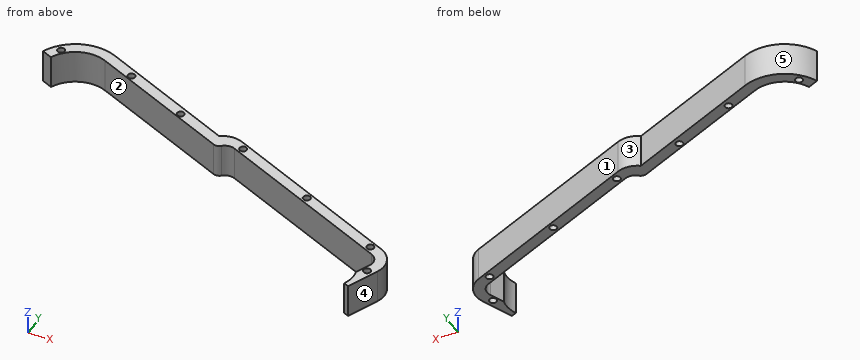
```python
from build123d import *

# Parameters (mm, degrees)
SKETCH1_R           = 14.25
SKETCH1_R_2         = 1.7
SKETCH1_R_3         = 1.6
BOSS_EXTRUDE1_DEPTH = 15
SKETCH5_R           = 1.25
SKETCH5_R_2         = 1.6
CUT_EXTRUDE4_DEPTH  = 16
CUT_EXTRUDE5_DEPTH  = 16
FILLET1_R           = 5
FILLET2_R           = 5
CUT_EXTRUDE6_DEPTH  = 16
CUT_EXTRUDE7_DEPTH  = 16
FILLET5_R           = 3
SKETCH9_R           = 14
CUT_EXTRUDE8_DEPTH  = 16


with BuildPart() as part:
    # Sketch1 → Boss-Extrude1 (new body)
    with BuildSketch(Plane.XY):
        with BuildLine():
            Line((-72.715301765, 90.837326721), (-152.817002247, 126.544575004))
            ThreePointArc((-152.817002247, 126.544575004), (-157.784388135, 127.370762315), (-162.524605276, 125.671394934))
            Line((-162.524605276, 125.671394934), (-222.299360222, 152.317421212))
            ThreePointArc((-222.299360222, 152.317421212), (-249.039738928, 142.066706765), (-238.78902448, 115.326328059))
            Line((-238.78902448, 115.326328059), (-179.014269534, 88.680301782))
            ThreePointArc((-179.014269534, 88.680301782), (-177.109561802, 84.018800254), (-173.174612442, 80.876558766))
            Line((-173.174612442, 80.876558766), (-93.072911961, 45.169310483))
            ThreePointArc((-93.072911961, 45.169310483), (-85.421957972, 44.965480094), (-79.867786674, 50.231391692))
            Line((-79.867786674, 50.231391692), (-67.653220557, 77.632201435))
            ThreePointArc((-67.653220557, 77.632201435), (-67.449390168, 85.283155423), (-72.715301765, 90.837326721))
        make_face()
        with Locations((-230.544192351, 133.821874636)):
            Circle(SKETCH1_R, mode=Mode.SUBTRACT)
        with Locations((-95.571468701, 49.02024728)):
            Circle(SKETCH1_R_2, mode=Mode.SUBTRACT)
        with Locations((-132.105881692, 65.306335437)):
            Circle(SKETCH1_R_2, mode=Mode.SUBTRACT)
        with Locations((-168.640294682, 81.592423593)):
            Circle(SKETCH1_R_2, mode=Mode.SUBTRACT)
        with Locations((-150.318445506, 122.693638207)):
            Circle(SKETCH1_R_3, mode=Mode.SUBTRACT)
        with Locations((-113.784032516, 106.407550051)):
            Circle(SKETCH1_R_3, mode=Mode.SUBTRACT)
        with Locations((-77.249619525, 90.121461895)):
            Circle(SKETCH1_R_3, mode=Mode.SUBTRACT)
        with Locations((-81.295075004, 54.152214057)):
            Circle(SKETCH1_R_2, mode=Mode.SUBTRACT)
        with Locations((-71.52342211, 76.072861852)):
            Circle(SKETCH1_R_3, mode=Mode.SUBTRACT)
        with Locations((-168.932649456, 106.357056211)):
            Circle(SKETCH1_R_2, mode=Mode.SUBTRACT)
    extrude(amount=BOSS_EXTRUDE1_DEPTH)

    # Sketch5 → Cut-Extrude4 (cut, through all)
    with BuildSketch(Plane.XY.offset(15)):
        with Locations((-196.466353254, 99.744559857)):
            Circle(SKETCH5_R)
        with Locations((-224.780523322, 112.366278179)):
            Circle(SKETCH5_R)
        with Locations((-210.733772287, 143.877209383)):
            Circle(SKETCH5_R_2)
        with Locations((-182.419602219, 131.255491062)):
            Circle(SKETCH5_R_2)
        with Locations((-242.947351213, 145.810375386)):
            Circle(SKETCH5_R_2)
        with Locations((-247.751623016, 135.033002179)):
            Circle(SKETCH5_R)
    extrude(amount=-CUT_EXTRUDE4_DEPTH, mode=Mode.SUBTRACT)

    # Sketch6 → Cut-Extrude5 (cut, through all)
    with BuildSketch(Plane.XY.offset(15)):
        Polygon((-158.059591703, 123.407293834), (-70.184261161, 84.234764078), (-86.470349317, 47.700351088), (-174.345679859, 86.872880843), align=None)
    extrude(amount=-CUT_EXTRUDE5_DEPTH, mode=Mode.SUBTRACT)

    # Fillet1
    fillet1_edges = [part.edges().sort_by_distance(p)[0] for p in [
        (-174.345679859, 86.872880843, 7.5),
        (-158.059591703, 123.407293834, 7.5),
    ]]
    fillet(fillet1_edges, radius=FILLET1_R)

    # Fillet2
    fillet2_edges = [part.edges().sort_by_distance(p)[0] for p in [
        (-70.184261161, 84.234764078, 7.5),
        (-86.470349317, 47.700351088, 7.5),
    ]]
    fillet(fillet2_edges, radius=FILLET2_R)

    # Sketch7 → Cut-Extrude6 (cut, through all)
    with BuildSketch(Plane.XY.offset(15)):
        Polygon((-249.039738928, 142.066706765), (-73.760503615, 63.931796563), (-92.871338518, 21.060658435), (-268.15057383, 99.195568636), align=None)
    extrude(amount=-CUT_EXTRUDE6_DEPTH, mode=Mode.SUBTRACT)

    # Sketch8 → Cut-Extrude7 (cut, through all)
    with BuildSketch(Plane.XY.offset(15)):
        with BuildLine():
            Line((-147.743052942, 113.607873768), (-224.335121242, 147.750619588))
            ThreePointArc((-224.335121242, 147.750619588), (-244.45553121, 140.069846398), (-236.831015973, 119.928050513))
            Line((-236.831015973, 119.928050513), (-160.324966884, 85.309789022))
            Line((-160.324966884, 85.309789022), (-147.743052942, 113.607873768))
        make_face()
    extrude(amount=-CUT_EXTRUDE7_DEPTH, mode=Mode.SUBTRACT)

    # Fillet5
    fillet5_edges = [part.edges().sort_by_distance(p)[0] for p in [
        (-159.987852597, 119.066285997, 7.5),
    ]]
    fillet(fillet5_edges, radius=FILLET5_R)

    # Sketch9 → Cut-Extrude8 (cut, through all)
    with BuildSketch(Plane.XY.offset(15)):
        with Locations((-88.728751121, 70.604250791)):
            Circle(SKETCH9_R)
    extrude(amount=-CUT_EXTRUDE8_DEPTH, mode=Mode.SUBTRACT)


solid = part.part
```
Work out the finished part from the listing and answer in its coordinate system (mm). Face numbers are marked on the shaded views. A direction names the side the tool comes from. Give positions to 0.01 mm unless a question says otherwise; leave off trailing zeros. Order: outer loops, then holes, each group sorted by start corner. A loop starts at its lowest first (then second) coordinate and runs counter-clockwise, first axis right, second up.
1. Section B-B, the plane y = 117.5 is taken. Determine the outline of the cut face in (x, z), and give its area (3 significant figures).
Result sheet:
outline: (-144.81, 0) - (-132.53, 0) - (-132.53, 15) - (-144.81, 15) - close
area: 184 mm2
2. Each of these flat-tipped pins is pushed along its axis until it touches: P1, Ø8, axis at x = -108.5, z = 9.5, coming from the +Y side; P2, Ø4, axis at y = 93, z = 6.5, coming from the -X side; P3, Ø2.5, axis at x = -150.32, y = 122.69, coming from the +Z side; P4, Ø2, axis at y = 143, z = 13, coming from the +X side. Where does it stop, or does it pass through?
Result sheet:
P1: stops at y = 108.57
P2: stops at x = -94.33
P3: passes through
P4: stops at x = -199.15
3. Section A-A, the plane z = 2.75 is taken. Determine the outline of the cut face in (x, y).
Result sheet:
outline: (-249.04, 142.07) - (-244.47, 140.03) arc R15.25 cw to (-224.34, 147.75) - (-162.1, 120.01) arc R3 ccw to (-158.87, 120.52) arc R5 cw to (-153.49, 121.37) - (-74.75, 86.27) arc R5 cw to (-72.22, 79.67) - (-75.01, 73.41) arc R14 cw to (-75.94, 64.9) - (-73.76, 63.93) - (-67.65, 77.63) arc R10 ccw to (-72.72, 90.84) - (-152.82, 126.54) arc R10 ccw to (-162.52, 125.67) - (-222.3, 152.32) arc R20.25 ccw to start; hole circle Ø3.2 at (-242.95, 145.81); hole circle Ø3.2 at (-210.73, 143.88); hole circle Ø3.2 at (-182.42, 131.26); hole circle Ø3.2 at (-150.32, 122.69); hole circle Ø3.2 at (-113.78, 106.41); hole circle Ø3.2 at (-77.25, 90.12); hole circle Ø3.2 at (-71.52, 76.07)
4. The mould has two halves that part along X. Classify the marked faces 3, 4 and 5: released by +X, released by -X, zero draft, split by the parting line, or undercut.
Result sheet:
face 3: undercut
face 4: released by +X
face 5: split by the parting line
5. For the marked faces 1 and 2, determine the directions among +Z, -Z, +X, -X, +Y, -Y from which every point of the face is accessible in a straight line to the end or side of a thin tool.
Result sheet:
face 1: +Z, -Z, +X, +Y
face 2: +Z, -Z, -Y
6. Section C-C, the plane x = -204.5 is taken. Determine the outline of the cut face in (y, z), and give its area (3 significant figures).
Result sheet:
outline: (138.91, 0) - (144.38, 0) - (144.38, 15) - (138.91, 15) - close
area: 82.1 mm2
7. Straight lines are drawn through the part: L1, parallel to X at y = 141.5, z = 10.5; L2, parallel to Y at x = -182, z = 12.75; L3, parallel to X at y = 107.5, z = 5. For each, find the intervals that lie inside material, in ascending order.
Result sheet:
L1: x = -247.77 to -243.72, -210.31 to -198.03
L2: y = 128.88 to 129.71, 132.8 to 134.35
L3: x = -122.37 to -114.95, -112.62 to -110.09
